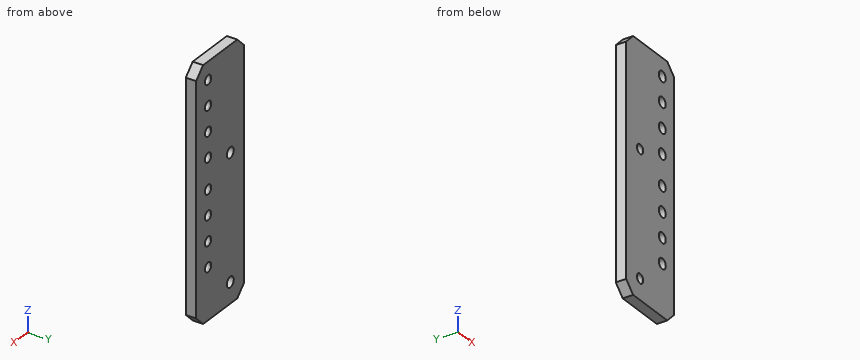
```python
from build123d import *

# Parameters (mm, degrees)
SKETCH1_W                                        = 34.5
SKETCH1_H                                        = 120
BOSS_EXTRUDE1_DEPTH                              = 5
CBORE_FOR_M4_HEX_HEAD_MACHINE_SCREW2_D           = 4.5
CBORE_FOR_M4_HEX_HEAD_MACHINE_SCREW2_DEPTH       = 12
CBORE_FOR_M4_HEX_HEAD_MACHINE_SCREW2_CBORE_D     = 5
CBORE_FOR_M4_HEX_HEAD_MACHINE_SCREW2_CBORE_DEPTH = 4.2
CBORE_FOR_M4_HEX_HEAD_MACHINE_SCREW2_TIP         = 1.351936393
CBORE_FOR_M4_HEX_HEAD_MACHINE_SCREW3_AT_COUNT    = 2
CBORE_FOR_M4_HEX_HEAD_MACHINE_SCREW3_AT_PITCH    = 50.8
LPATTERN1_COUNT                                  = 4
LPATTERN1_PITCH                                  = 12
CHAMFER1_SIZE                                    = 5


with BuildPart() as part:
    # Sketch1 → Boss-Extrude1 (new body)
    with BuildSketch(Plane(origin=(0, 0, 0), x_dir=(1, 0, 0), z_dir=(0, 1, 0))):
        Rectangle(SKETCH1_W, SKETCH1_H)
    extrude(amount=BOSS_EXTRUDE1_DEPTH)

    # CBORE for M4 Hex Head Machine Screw2
    with Locations(Plane(origin=(0, 5, 0), x_dir=(1, 0, 0), z_dir=(0, 1, 0))):
        with Locations((-7.25, 50), (-7.25, -10)):
            CounterBoreHole(CBORE_FOR_M4_HEX_HEAD_MACHINE_SCREW2_D / 2, CBORE_FOR_M4_HEX_HEAD_MACHINE_SCREW2_CBORE_D / 2, CBORE_FOR_M4_HEX_HEAD_MACHINE_SCREW2_CBORE_DEPTH, depth=CBORE_FOR_M4_HEX_HEAD_MACHINE_SCREW2_DEPTH)
            with Locations((0, 0, -(CBORE_FOR_M4_HEX_HEAD_MACHINE_SCREW2_DEPTH + CBORE_FOR_M4_HEX_HEAD_MACHINE_SCREW2_TIP / 2))):  # 118° drill point
                Cone(0, CBORE_FOR_M4_HEX_HEAD_MACHINE_SCREW2_D / 2, CBORE_FOR_M4_HEX_HEAD_MACHINE_SCREW2_TIP, mode=Mode.SUBTRACT)

    # Sketch6 → CBORE for M4 Hex Head Machine Screw3 (revolve, cut)
    with BuildSketch(Plane(origin=(8.672, 0, -35.4), x_dir=(0, 0, -1), z_dir=(1, 0, 0))):
        Polygon((0, 0), (0, 13.351936393), (2.25, 12), (2.25, 4.2), (2.5, 4.2), (2.5, 0), align=None)
    cbore_for_m4_hex_head_machine_screw3 = revolve(axis=Axis((8.672, -6.35, -35.4), (0, 1, 0)), mode=Mode.SUBTRACT)

    # CBORE for M4 Hex Head Machine Screw3 at: CBORE for M4 Hex Head Machine Screw3 ×2
    with Locations(*[(0, 0, i * CBORE_FOR_M4_HEX_HEAD_MACHINE_SCREW3_AT_PITCH) for i in range(1, CBORE_FOR_M4_HEX_HEAD_MACHINE_SCREW3_AT_COUNT)]):
        add(cbore_for_m4_hex_head_machine_screw3, mode=Mode.SUBTRACT)

    # LPattern1: CBORE for M4 Hex Head Machine Screw3 ×4
    with Locations(*[(0, 0, i * LPATTERN1_PITCH) for i in range(1, LPATTERN1_COUNT)]):
        add(cbore_for_m4_hex_head_machine_screw3, mode=Mode.SUBTRACT)

    # LPattern1 copy 1 sketch → LPattern1 copy 1 (revolve, cut)
    with BuildSketch(Plane(origin=(8.672, 0, 27.4), x_dir=(0, 0, -1), z_dir=(1, 0, 0))):
        Polygon((0, 0), (0, 13.351936393), (2.25, 12), (2.25, 4.2), (2.5, 4.2), (2.5, 0), align=None)
    revolve(axis=Axis((8.672, -6.35, 27.4), (0, 1, 0)), mode=Mode.SUBTRACT)

    # LPattern1 copy 2 sketch → LPattern1 copy 2 (revolve, cut)
    with BuildSketch(Plane(origin=(8.672, 0, 39.4), x_dir=(0, 0, -1), z_dir=(1, 0, 0))):
        Polygon((0, 0), (0, 13.351936393), (2.25, 12), (2.25, 4.2), (2.5, 4.2), (2.5, 0), align=None)
    revolve(axis=Axis((8.672, -6.35, 39.4), (0, 1, 0)), mode=Mode.SUBTRACT)

    # LPattern1 copy 3 sketch → LPattern1 copy 3 (revolve, cut)
    with BuildSketch(Plane(origin=(8.672, 0, 51.4), x_dir=(0, 0, -1), z_dir=(1, 0, 0))):
        Polygon((0, 0), (0, 13.351936393), (2.25, 12), (2.25, 4.2), (2.5, 4.2), (2.5, 0), align=None)
    revolve(axis=Axis((8.672, -6.35, 51.4), (0, 1, 0)), mode=Mode.SUBTRACT)

    # Chamfer1
    chamfer1_edges = [part.edges().sort_by_distance(p)[0] for p in [
        (17.25, 2.5, 60),
        (-17.25, 2.5, 60),
        (-17.25, 2.5, -60),
        (17.25, 2.5, -60),
    ]]
    chamfer(chamfer1_edges, length=CHAMFER1_SIZE)


solid = part.part
```
For this review, take the finished solid that the model builds, in its own axes (mm). Coordinates: 2 decimals unless noted, no trailing zeros. Write each loop counter-clockwise with the first axis right and the second up, starting at its lowest first coordinate (ties: lowest second). Pieces come first, ordered by that corner, then holes. Notation, with made-up numbers: (8, 34.5) - (60, 34.5) arc R21 ccw to (60, 72.5) - close; hole circle Ø4 at (1, 76). An arc over 180 degrees is marked (long way). Put each result on its own line as item: value.
1. Add section B-B, the plane x = -7.25. Give the boundary of the cut face in (y, z), then the cut area to 3 significant figures.
Values found:
outline: (0, -60) - (5, -60) - (5, -52.5) - (0.8, -52.5) - (0.8, -52.25) - (0, -52.25) - close; (0, -47.75) - (0.8, -47.75) - (0.8, -47.5) - (5, -47.5) - (5, 7.5) - (0.8, 7.5) - (0.8, 7.75) - (0, 7.75) - close; (0, 12.25) - (0.8, 12.25) - (0.8, 12.5) - (5, 12.5) - (5, 60) - (0, 60) - close
area: 551 mm²
2. Add section A-A, the plane z = 39.4. Give the boundary of the cut face in (x, y).
Values found:
outline: (-17.25, 0) - (6.17, 0) - (6.17, 4.2) - (6.42, 4.2) - (6.42, 5) - (-17.25, 5) - close; (10.92, 4.2) - (11.17, 4.2) - (11.17, 0) - (17.25, 0) - (17.25, 5) - (10.92, 5) - close
3. Add section C-C, the plane y = 2.6. Count the separate pieces of the cut face and the enclosed holes in it, then the cut area to 3 significant figures.
Values found:
separate pieces: 1
enclosed holes: 10
area: 3,890 mm²
4. Wall thickness on probe 1 along X at (y, z) = (2.4, -23.4); probe 2 along X at (y, z) = (0.2, -50); probe 3 along Z at (x, y) = (-7.25, 2.9): over which ranges is each line inside the solid? List them lowest first.
Values found:
probe 1: -17.25 to 6.17, 11.17 to 17.25
probe 2: -17.25 to -9.5, -5 to 17.25
probe 3: -60 to -52.5, -47.5 to 7.5, 12.5 to 60
5. Add section D-D, the plane x = -15. Give the boundary of the cut face in (y, z), then the cut area to 4 significant figures.
Values found:
outline: (0, -57.25) - (5, -57.25) - (5, 57.25) - (0, 57.25) - close
area: 572.5 mm²
